from build123d import *

# Parameters (mm, degrees)
EXTRUDE_1_DEPTH     = 19.8
EXTRUDE_1_2_DEPTH   = 19.8
SKETCH_2_W          = 1
SKETCH_2_H          = 0.8
CUT_EXTRUDE_1_DEPTH = 8
EXTRUDE_2_DEPTH     = 8.5
EXTRUDE_3_DEPTH     = 8.5
CUT_EXTRUDE_2_REACH = 72.966
SKETCH_5_R          = 1.9
CUT_EXTRUDE_5_REACH = 68.083
SKETCH_8_W          = 19.8
SKETCH_8_H          = 8.5
SKETCH_9_R          = 1.65
EXTRUDE_4_DEPTH     = 11.3
CUT_EXTRUDE_6_REACH = 72.966
SKETCH_10_R         = 2


with BuildPart() as part:
    # Sketch 1 → Extrude 1 (new body)
    with BuildSketch(Plane.XY):
        Polygon((-40.673096552, 29.7), (-40.673096552, 2.8), (-48.673096552, 2.8), (-48.673096552, 34.7), (-41.673096552, 34.7), (-0.073096552, 34.7), (-0.073096552, 29.7), align=None)
    extrude(amount=EXTRUDE_1_DEPTH)



with BuildPart() as body_2:
    # Sketch 1 → Extrude 1 2 (new body)
    with BuildSketch(Plane.XY):
        Polygon((-48.673096552, -8.5), (-40.673096552, -8.5), (-40.673096552, -3.2), (-40.673096552, 0), (-48.673096552, 0), align=None)
    extrude(amount=EXTRUDE_1_2_DEPTH)

    # Sketch 2 → Cut-Extrude 1 (cut)
    with BuildSketch(Plane.ZY.offset(48.673096552)):
        with Locations((9.9, -0.4)):
            Rectangle(SKETCH_2_W, SKETCH_2_H)
    extrude(amount=-CUT_EXTRUDE_1_DEPTH, mode=Mode.SUBTRACT)


with BuildPart() as part_1:
    add(part.part)

    add(body_2.part)  # Extrude 2 merges body 2
    # Sketch 3 → Extrude 2 (add)
    with BuildSketch(Plane.XY.offset(19.8)):
        Polygon((-48.673096552, -8.5), (-32.173096552, -8.5), (-0.073096552, 29.7), (-0.073096552, 34.7), (-48.673096552, 34.7), align=None)
    extrude(amount=EXTRUDE_2_DEPTH)

    # Sketch 4 → Extrude 3 (add)
    with BuildSketch(Plane(origin=(0, 0, 0), x_dir=(-1, 0, 0), z_dir=(0, 0, -1))):
        Polygon((48.673096552, -8.5), (48.673096552, 34.7), (0.073096552, 34.7), (0.073096552, 29.7), (32.173096552, -8.5), align=None)
    extrude(amount=EXTRUDE_3_DEPTH)

    # Sketch 5 → Cut-Extrude 2 (cut, up to next)
    with BuildSketch(Plane(origin=(0, 34.7, 0), x_dir=(1, 0, 0), z_dir=(0, 1, 0)), mode=Mode.PRIVATE) as cut_extrude_2_sk1:
        with Locations(Location((-10.073096552, -9.9, 0), (0, 0, 270))):
            Circle(SKETCH_5_R)
    cut_extrude_2_tool1 = extrude(cut_extrude_2_sk1.sketch, amount=-CUT_EXTRUDE_2_REACH, mode=Mode.PRIVATE) & part_1.part
    add(cut_extrude_2_tool1.solids().sort_by_distance((-10.073097, 34.7, 9.9))[0], mode=Mode.SUBTRACT)

    # Cut-Extrude 5: up to this plane
    cut_extrude_5_end = Plane(origin=(-0.073096552, 29.7, -8.5), z_dir=(-0.7655864074982082, 0.6433330806464003, 0))
    # Sketch 8 → Cut-Extrude 5 (cut, up to the surface)
    with BuildSketch(Plane.ZY.offset(48.673096552), mode=Mode.PRIVATE) as cut_extrude_5_sk1:
        with Locations((9.9, -4.25)):
            Rectangle(SKETCH_8_W, SKETCH_8_H)
    cut_extrude_5_tool1 = split(extrude(cut_extrude_5_sk1.sketch, amount=-CUT_EXTRUDE_5_REACH, mode=Mode.PRIVATE), bisect_by=cut_extrude_5_end, keep=Keep.BOTH, mode=Mode.PRIVATE)
    add(cut_extrude_5_tool1.solids().sort_by_distance((-48.673097, -4.25, 9.9))[0], mode=Mode.SUBTRACT)

    # Sketch 9 → Extrude 4 (add)
    with BuildSketch(Plane.XZ.offset(-2.8)):
        with Locations(Location((-45.273096552, 14.9, 0), (0, 0, 90))):
            Circle(SKETCH_9_R)
        with Locations(Location((-45.273096552, 4.9, 0), (0, 0, 90))):
            Circle(SKETCH_9_R)
    extrude(amount=EXTRUDE_4_DEPTH)

    # Sketch 10 → Cut-Extrude 6 (cut, up to next)
    with BuildSketch(Plane(origin=(0, -8.5, 0), x_dir=(-1, 0, 0), z_dir=(0, -1, 0)), mode=Mode.PRIVATE) as cut_extrude_6_sk1:
        with Locations(Location((40.677003756, -24.3, 0), (0, 0, 90))):
            Circle(SKETCH_10_R)
    cut_extrude_6_tool1 = extrude(cut_extrude_6_sk1.sketch, amount=-CUT_EXTRUDE_6_REACH, mode=Mode.PRIVATE) & part_1.part
    # Sketch 10 → Cut-Extrude 6 (cut, up to next)
    with BuildSketch(Plane(origin=(0, -8.5, 0), x_dir=(-1, 0, 0), z_dir=(0, -1, 0)), mode=Mode.PRIVATE) as cut_extrude_6_sk2:
        with Locations(Location((40.673096552, 4.495764624, 0), (0, 0, 90))):
            Circle(SKETCH_10_R)
    cut_extrude_6_tool2 = extrude(cut_extrude_6_sk2.sketch, amount=-CUT_EXTRUDE_6_REACH, mode=Mode.PRIVATE) & part_1.part
    add(cut_extrude_6_tool1.solids().sort_by_distance((-40.677004, -8.5, 24.3))[0], mode=Mode.SUBTRACT)
    add(cut_extrude_6_tool2.solids().sort_by_distance((-40.673097, -8.5, -4.495765))[0], mode=Mode.SUBTRACT)


solid = part_1.part
Can you work these out from the model? Positions are in its coordinate system, mm. A direction names the side the tool comes from. Coordinates: 2 decimals unless noted, no trailing zeros. Loops run counter-clockwise (first coordinate to the right, second up) from the corner with the lowest first, then second, coordinate; pieces in that order, holes last. Notation, with made-up numbers: M 79.5,77 L 111.5,77 A20 cw 111.5,87 Z; hole C -39,3 d10. An arc over 180 degrees is marked long. Return JSON: item names as keys, results as strings. Group by question number.
Item 1: Imagine slicing it at D-D (x = -36). Please give me the cut outline in (y, z).
Item 2: On a 3-axis mill with a long thin cutter (end or side, diameter ignored), from which of +Z, -Z, +X, -X, +Y, -Y can I reach the whole of each face in a straight line? I mean faces 4 (the flat face through (-38, -8.5, 24)), 5 (the flat face through (-30, 15, 19.8)). Say none if no direction works.
Item 3: If I drill on L1, parallel to Z at x = -11.5, y = 20.5; L2, parallel to X at y = 32.4, z = 9.9; L3, parallel to Z at x = -39, y = 16, over which ranges is the centre line in solid material (lowest first)? Write a range as from..to.
Item 4: Imagine slicing it at C-C (z = 14.9). Please give me the cut outline in (x, y).
Item 5: I'm going to push flat-ended pins straight in: pin 1 Ø1.5 at (x, z) = (-21.5, 8) entering from -Y; pin 2 Ø5 at (y, z) = (17, 16) entering from +X; pin 3 Ø1.5 at (y, z) = (0, 17) entering from +X; pin 4 Ø2.5 at (x, z) = (-40.68, 24.3) entering from +Y. Where does each tip first touch, or does it pass through?
Item 6: Imagine slicing it at B-B (z = 9.9). Please give me the cut outline in (x, y).
Item 7: Imagine slicing it at A-A (y = -2). Please give me the cut outline in (x, z), and give its area (3 significant figures).
Item 8: Thinking about a two-plate mould opening in X: for faces 1 (the cylindrical face through (-46.664, -2.771, 5.787)), 2 (the flat face through (-45, -8.5, 15)), 3 (the cylindrical face through (-42.451, 12.798, 23.377)), which applies, released by +X, released by -X, zero draft, split by the parting line, or undercut?
Verdict:
{
 "1": {"outline": "M -8.5,-8.5 L 34.7,-8.5 L 34.7,28.3 L -8.5,28.3 L -8.5,19.8 L 29.7,19.8 L 29.7,0 L -8.5,0 Z"},
 "2": {"face 4": "+Z, -Z, +X, -X, -Y", "face 5": "+X, -Y"},
 "3": {"L1": "z = -8.5..0, 19.8..28.3", "L2": "x = -48.67..-11.97, -8.17..-0.07", "L3": "z = -8.5..-5.59, -3.4..0, 19.8..23.21, 25.39..28.3"},
 "4": {"outline": "M -48.67,2.8 L -46.92,2.8 L -46.92,-8.5 L -43.62,-8.5 L -43.62,2.8 L -40.67,2.8 L -40.67,29.7 L -0.07,29.7 L -0.07,34.7 L -48.67,34.7 Z"},
 "5": {"pin 1": "stops at y = 29.7", "pin 2": "stops at x = -40.67", "pin 3": "stops at x = -44.32", "pin 4": "passes through"},
 "6": {"outline": "M -48.67,2.8 L -40.67,2.8 L -40.67,29.7 L -11.97,29.7 L -11.97,34.7 L -48.67,34.7 Z; M -8.17,29.7 L -0.07,29.7 L -0.07,34.7 L -8.17,34.7 Z"},
 "7": {"outline": "M -48.67,-8.5 L -26.71,-8.5 L -26.71,0 L -48.67,0 Z; M -48.67,19.8 L -26.71,19.8 L -26.71,28.3 L -48.67,28.3 Z; C -45.27,4.9 d3.3; C -45.27,14.9 d3.3; hole C -40.68,24.3 d4; hole C -40.67,-4.5 d4", "area": "365 mm^2"},
 "8": {"face 1": "split by the parting line", "face 2": "zero draft", "face 3": "undercut"}
}
